Geometry: final body of the model. Coordinates: model frame, mm. A direction names the side the tool comes from. Coordinates: 2 decimals unless noted, no trailing zeros. Order: outer loops, then holes, each group sorted by start corner. A loop starts at its lowest first (then second) coordinate and runs counter-clockwise, first axis right, second up. Notation, with made-up numbers: M 1.5,80.25 L 39.5,80.25 A27 cw 39.5,96.25 Z; hole C 77,60 d5. An arc over 180 degrees is marked long. Use CSV: the item, a comma, the result in double quotes. Start each with the question number.
1. Pull-direction query (Z, two-part tool) for faces 1 (the conical face through (3.348, -0.285, 10.797)), 2 (the flat face through (-1.42, -1.232, 9.914)), 3 (the flat face through (1.38, -1.232, 9.936)), 4 (the cylindrical face through (-3.859, -2.268, -11.297)); classes: pulls with the +Z half, pulls with the -Z half, needs draft (parallel to the pull), parting line crosses it, or undercut.
2. Set-up query: faces 5 (the flat face through (0, -0.5, 12)), 6 (the flat face through (-2.8, -1, -8)). Return all of +Z, -Z, +X, -X, +Y, -Y with unobstructed straight access to the full face (end or side cutting, diameter ignored); none if empty.
3. Section query C-C on y = -3.05. Return the cut outline in (x, z), and give its area (3 significant figures).
4. Material intervals for line 1 (Z direction, x = 0.5, y = -1.45); line 2 (Y direction, x = -0.25, z = 4.75); line 3 (X direction, y = -1.6, z = -6.25), sorted ascending.
5. Section query A-A on z = -7.5. Return the cut outline in (x, y).
6. First-contact query: P1, Ø2, axis at x = 2, y = -0.5, coming from the +Z side; P2, Ø1, axis at x = 2, z = 0.5, coming from the -Y side; P3, Ø4.5, axis at x = 1, z = 6, coming from the +Y side; P4, Ø1.5, axis at x = -0.5, z = -3, coming from the -Y side. Flat tips, straight axial feed; report the tip coordinate or a pass-through.
7. Section query D-D on z = -1.25. Return the cut outline in (x, y).
8. Section query B-B on y = -1.7. Return the cut outline in (x, z).
from build123d import *

# Parameters (mm, degrees)
F0_W     = 10
F0_H     = 25
F1_DEPTH = 2.5
F2_W     = 10
F2_H     = 25
F2_R     = 1.5
F3_DEPTH = 1
F4_R     = 10
F5_DEPTH = 25
F6_R     = 4
F7_SIZE  = 1


with BuildPart() as f1:
    # F0 (on Front) → F1 (new body)
    with BuildSketch(Plane.XZ):
        Rectangle(F0_W, F0_H)
        Polygon((0, -4.266838), (2.8, -5.883419), (2.8, -9.116581), (0, -10.733162), (-2.8, -9.116581), (-2.8, -5.883419), align=None, mode=Mode.SUBTRACT)
        Polygon((2.8, 5.883419), (0, 4.266838), (-2.8, 5.883419), (-2.8, 9.116581), (0, 10.733162), (2.8, 9.116581), align=None, mode=Mode.SUBTRACT)
    extrude(amount=F1_DEPTH)

    # F2 (on face) → F3 (join)
    with BuildSketch(Plane.XZ.offset(2.5)):
        Rectangle(F2_W, F2_H)
        Polygon((-2.8, -5.883419), (0, -4.266838), (2.8, -5.883419), (2.8, -9.116581), (0, -10.733162), (-2.8, -9.116581), align=None, mode=Mode.SUBTRACT)
        Polygon((-2.8, 9.116581), (0, 10.733162), (2.8, 9.116581), (2.8, 5.883419), (0, 4.266838), (-2.8, 5.883419), align=None, mode=Mode.SUBTRACT)
        Polygon((2.8, 9.116581), (0, 10.733162), (-2.8, 9.116581), (-2.8, 5.883419), (0, 4.266838), (2.8, 5.883419), align=None)
        with Locations((0, 7.5)):
            Circle(F2_R, mode=Mode.SUBTRACT)
        Polygon((2.8, -5.883419), (0, -4.266838), (-2.8, -5.883419), (-2.8, -9.116581), (0, -10.733162), (2.8, -9.116581), align=None)
        with Locations((0, -7.5)):
            Circle(F2_R, mode=Mode.SUBTRACT)
    extrude(amount=F3_DEPTH)

    # F4 (on face) → F5 (cut)
    with BuildSketch(Plane.YZ.offset(5)):
        with Locations((-12.5, 0)):
            Circle(F4_R)
    extrude(amount=-F5_DEPTH, mode=Mode.SUBTRACT)

    # F6
    f6_edges = [f1.edges().sort_by_distance(p)[0] for p in [
        (5, -1.75, 12.5),
        (-5, -1.75, 12.5),
        (-5, -1.75, -12.5),
        (5, -1.75, -12.5),
    ]]
    fillet(f6_edges, radius=F6_R)

    # F7
    f7_edges = [f1.edges().sort_by_distance(p)[0] for p in [
        (5, 0, 0),
    ]]
    chamfer(f7_edges, length=F7_SIZE)


solid = f1.part
Results list:
1,face 1,"pulls with the +Z half"
1,face 2,"undercut"
1,face 3,"undercut"
1,face 4,"pulls with the -Z half"
2,face 5,"+Z, +X, -X, +Y"
2,face 6,"+Y"
3,outline,"M -5,-8.5 A4 ccw -1,-12.5 L 1,-12.5 A4 ccw 5,-8.5 L 5,-3.27 L -5,-3.27 Z; M -5,3.27 L 5,3.27 L 5,8.5 A4 ccw 1,12.5 L -1,12.5 A4 ccw -5,8.5 Z; hole C 0,-7.5 d3; hole C 0,7.5 d3"
3,area,"157 mm²"
4,line 1,"z = -12.5 to -10.44, -4.56 to 4.56, 10.44 to 12.5"
4,line 2,"y = -3.5 to -2.5"
4,line 3,"x = -5 to -2.8, 2.8 to 5"
5,outline,"M -5,-3.5 L -1.5,-3.5 L -1.5,-2.5 L -2.8,-2.5 L -2.8,0 L -4,0 L -5,-1 Z; M 1.5,-3.5 L 5,-3.5 L 5,-1 L 4,0 L 2.8,0 L 2.8,-2.5 L 1.5,-2.5 Z"
6,P1,"stops at z = 12.5"
6,P2,"stops at y = -2.55"
6,P3,"stops at y = 0"
6,P4,"stops at y = -3.23"
7,outline,"M -5,-2.58 L 5,-2.58 L 5,-1 L 4,0 L -4,0 L -5,-1 Z"
8,outline,"M -5,-8.5 A4 ccw -1,-12.5 L 1,-12.5 A4 ccw 5,-8.5 L 5,8.5 A4 ccw 1,12.5 L -1,12.5 A4 ccw -5,8.5 Z; hole M -2.8,-9.12 L 0,-10.73 L 2.8,-9.12 L 2.8,-5.88 L 0,-4.27 L -2.8,-5.88 Z; hole M -2.8,5.88 L 0,4.27 L 2.8,5.88 L 2.8,9.12 L 0,10.73 L -2.8,9.12 Z"
